Could you check a few things on this model? Use its own coordinates, in mm. Face numbers are marked on the shaded views. A direction names the side the tool comes from. Give positions to 0.01 mm unless a question says otherwise; leave off trailing zeros. Order: outer loops, then holes, each group sorted by start corner. A loop starts at its lowest first (then second) coordinate and runs counter-clockwise, first axis right, second up. Notation, with made-up numbers: (60, -2) -> (68, -2) arc R29 ccw to (68, 21) -> close; hole circle Ø4 at (26.5, 1.25). An arc over 180 degrees is marked (long way). One line per item, written item: value.
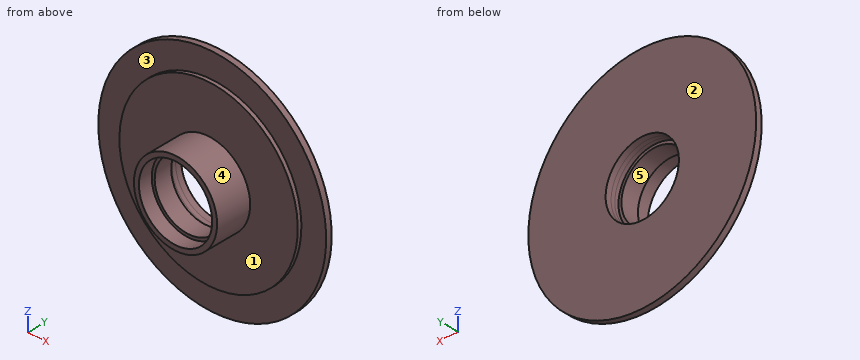
```python
from build123d import *
from build123d.topology import SkipClean

# Parameters (mm, degrees)
SKETCH1_R           = 57.5
SKETCH1_R_2         = 18.5
BOSS_EXTRUDE1_DEPTH = 3
BOSS_EXTRUDE2_START = 2
SKETCH2_R           = 45
SKETCH2_R_2         = 18.5
BOSS_EXTRUDE2_DEPTH = 2
BOSS_EXTRUDE3_START = 18
SKETCH3_R           = 21
SKETCH3_R_2         = 18.5
BOSS_EXTRUDE3_DEPTH = 18
BOSS_EXTRUDE4_START = -7
SKETCH4_R           = 18.5
SKETCH4_R_2         = 17
BOSS_EXTRUDE4_DEPTH = 9


with BuildPart() as part:
    # Sketch1 → Boss-Extrude1 (new body)
    with BuildSketch(Plane(origin=(0, 0, 0), x_dir=(1, 0, 0), z_dir=(0, 1, 0))):
        with Locations(Location((0, 0, 0), (0, 0, 270))):
            Circle(SKETCH1_R)
        with Locations(Location((0, 0, 0), (0, 0, 270))):
            Circle(SKETCH1_R_2, mode=Mode.SUBTRACT)
    extrude(amount=BOSS_EXTRUDE1_DEPTH)

    # Sketch2 → Boss-Extrude2 (add)
    with SkipClean():  # the faces are left unmerged after this step: merging them gives an invalid solid
        with BuildSketch(Plane.XZ.offset(BOSS_EXTRUDE2_START)):
            with Locations(Location((0, 0, 0), (0, 0, 270))):
                Circle(SKETCH2_R)
            with Locations(Location((0, 0, 0), (0, 0, 270))):
                Circle(SKETCH2_R_2, mode=Mode.SUBTRACT)
        extrude(amount=-BOSS_EXTRUDE2_DEPTH)

    # Sketch3 → Boss-Extrude3 (add)
    with SkipClean():  # the faces are left unmerged after this step: merging them gives an invalid solid
        with BuildSketch(Plane.XZ.offset(2).offset(BOSS_EXTRUDE3_START)):
            with Locations(Location((0, 0, 0), (0, 0, 270))):
                Circle(SKETCH3_R)
            with Locations(Location((0, 0, 0), (0, 0, 270))):
                Circle(SKETCH3_R_2, mode=Mode.SUBTRACT)
        extrude(amount=-BOSS_EXTRUDE3_DEPTH)

    # Sketch4 → Boss-Extrude4 (add)
    with SkipClean():  # the faces are left unmerged after this step: merging them gives an invalid solid
        with BuildSketch(Plane.XZ.offset(20).offset(BOSS_EXTRUDE4_START)):
            with Locations(Location((0, 0, 0), (0, 0, 270))):
                Circle(SKETCH4_R)
            with Locations(Location((0, 0, 0), (0, 0, 270))):
                Circle(SKETCH4_R_2, mode=Mode.SUBTRACT)
        extrude(amount=-BOSS_EXTRUDE4_DEPTH)


solid = part.part
```
1) For P1, Ø11, axis at x = -3.5, z = 9, coming from the -Y side; P2, Ø10, axis at x = 18, y = 0.5, coming from the -Z side; P3, Ø12, axis at x = 41, y = -1, coming from the +Z side; P4, Ø6, axis at x = 12, y = 0.5, coming from the +Z side, each with a flat end and sliding along its axis, tell me the tip position at first contact or that it passes through.
Answer below:
P1: passes through
P2: stops at z = -56.01
P3: stops at z = 45.56
P4: stops at z = 56.79
2) Suppose I cut it at B-B, the plane z = 0. Write out the boundary of the cut face in (x, y).
Answer below:
outline: (-57.5, 0) -> (-45, 0) -> (-45, -2) -> (-21, -2) -> (-21, -20) -> (-18.5, -20) -> (-18.5, -13) -> (-17, -13) -> (-17, -4) -> (-18.5, -4) -> (-18.5, 3) -> (-57.5, 3) -> close; (17, -13) -> (18.5, -13) -> (18.5, -20) -> (21, -20) -> (21, -2) -> (45, -2) -> (45, 0) -> (57.5, 0) -> (57.5, 3) -> (18.5, 3) -> (18.5, -4) -> (17, -4) -> close
3) Suppose I cut it at D-D, the plane z = -22.5. Write out the boundary of the cut face in (x, y).
Answer below:
outline: (-52.92, 0) -> (-38.97, 0) -> (-38.97, -2) -> (38.97, -2) -> (38.97, 0) -> (52.92, 0) -> (52.92, 3) -> (-52.92, 3) -> close
4) Suppose I cut it at C-C, the plane y = -8. Write out the boundary of the cut face in (x, z), then the cut area to 3 significant figures.
Answer below:
outline: circle Ø42 at (0, 0); hole circle Ø34 at (0, 0)
area: 478 mm2
5) Suppose I cut it at A-A, the plane x = 0. Write out the boundary of the cut face in (y, z), then the cut area to 3 significant figures.
Answer below:
outline: (-20, -21) -> (-2, -21) -> (-2, -45) -> (0, -45) -> (0, -57.5) -> (3, -57.5) -> (3, -18.5) -> (-4, -18.5) -> (-4, -17) -> (-13, -17) -> (-13, -18.5) -> (-20, -18.5) -> close; (-20, 18.5) -> (-13, 18.5) -> (-13, 17) -> (-4, 17) -> (-4, 18.5) -> (3, 18.5) -> (3, 57.5) -> (0, 57.5) -> (0, 45) -> (-2, 45) -> (-2, 21) -> (-20, 21) -> close
area: 457 mm2
6) For the marked faces 1 and 2, which set-ups out of +Z, -Z, +X, -X, +Y, -Y let a thin tool reach every point of the face, with its end or its side?
Answer below:
face 1: -Y
face 2: +Z, -Z, +X, -X, +Y
7) If I drill on line 1 along X through (y, z) = (1.6, 0); line 2 along X through (y, z) = (-1.2, 0); line 3 along Y through (x, z) = (25.5, -33.5), over which ranges is the centre line in solid material (lowest first)?
Answer below:
line 1: x = -57.5 to -18.5, 18.5 to 57.5
line 2: x = -45 to -18.5, 18.5 to 45
line 3: y = -2 to 3
8) We'd pull the mould along Z, two halves only. Please class the marked faces 3, 4 and 5: +Z half, -Z half, draft (parallel to the pull), parting line (faces both ways), or undercut.
Answer below:
face 3: draft
face 4: parting line
face 5: undercut
